Source: CAD feature listing. Evaluate the final solid. Frame: model axes, mm. Face numbers are marked on the shaded views. A direction names the side the tool comes from. Round coordinates to 2 decimals unless told otherwise and drop trailing zeros. Loops run counter-clockwise (first coordinate to the right, second up) from the corner with the lowest first, then second, coordinate; pieces in that order, holes last. Notation, with made-up numbers: (-3.75, 52.5) - (30.25, 52.5) arc R17 cw to (30.25, 63.5) - close; hole circle Ø7 at (-7, 50.25). An arc over 180 degrees is marked (long way). Write item = value, one per line. Start each with the question number.
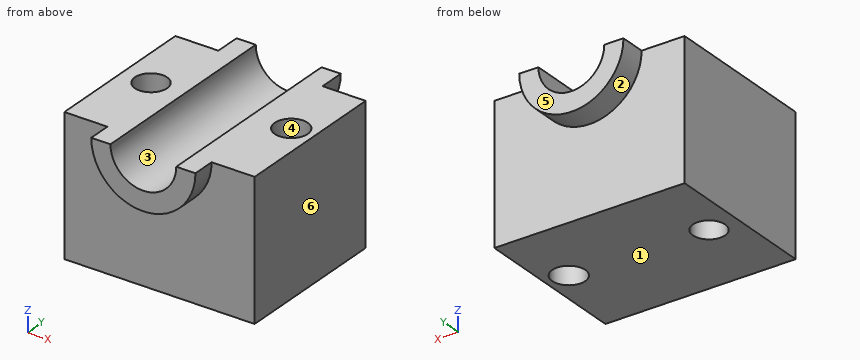
from build123d import *

# Parameters (mm, degrees)
F0_W     = 105.5908799171
F0_H     = 87.321691215
F1_DEPTH = 76.2
F3_DEPTH = 101.6
F4_DEPTH = 12.7
F5_DEPTH = 127
F6_R     = 8.9460405917
F7_DEPTH = 101.6
F6_R_2   = 9.1609397995
F8_DEPTH = 127


with BuildPart() as f1:
    # F0 (on Top) → F1 (new body)
    with BuildSketch(Plane.XY):
        with Locations((3.3811926842, 4.9695521593)):
            Rectangle(F0_W, F0_H)
    extrude(amount=F1_DEPTH)

    # F2 (on face) → F3 (join)
    with BuildSketch(Plane.XZ.offset(38.6912934482)):
        with BuildLine():
            ThreePointArc((-14.8835639872, 76.2), (3.3811926842, 57.9352433286), (21.6459493555, 76.2))
            Line((21.6459493555, 76.2), (-14.8835639872, 76.2))
        make_face()
        with BuildLine():
            ThreePointArc((-25.5366911298, 76.2), (3.3811926842, 47.282116186), (32.2990764981, 76.2))
            Line((32.2990764981, 76.2), (21.6459493555, 76.2))
            ThreePointArc((21.6459493555, 76.2), (3.3811926842, 57.9352433286), (-14.8835639872, 76.2))
            Line((-14.8835639872, 76.2), (-25.5366911298, 76.2))
        make_face()
    extrude(amount=-F3_DEPTH)

    # F2 (on face) → F4 (join)
    with BuildSketch(Plane.XZ.offset(38.6912934482)):
        with BuildLine():
            ThreePointArc((-25.5366911298, 76.2), (3.3811926842, 47.282116186), (32.2990764981, 76.2))
            Line((32.2990764981, 76.2), (21.6459493555, 76.2))
            ThreePointArc((21.6459493555, 76.2), (3.3811926842, 57.9352433286), (-14.8835639872, 76.2))
            Line((-14.8835639872, 76.2), (-25.5366911298, 76.2))
        make_face()
    extrude(amount=F4_DEPTH)

    # F5 (cut): a face of the model
    f5_faces = [f1.faces().sort_by_distance(p)[0] for p in [
        (3.3811926842, -38.6912934482, 68.4481965103),
    ]]
    extrude(f5_faces, amount=-F5_DEPTH, mode=Mode.SUBTRACT)

    # F6 (on face) → F7 (cut)
    with BuildSketch(Plane.XY.offset(76.2)):
        with Locations((-33.1366732717, 6.3863405958)):
            Circle(F6_R)
    extrude(amount=-F7_DEPTH, mode=Mode.SUBTRACT)

    # F6 (on face) → F8 (cut)
    with BuildSketch(Plane.XY.offset(76.2)):
        with Locations((43.499417603, 8.0732982606)):
            Circle(F6_R_2)
    extrude(amount=-F8_DEPTH, mode=Mode.SUBTRACT)


solid = f1.part
(1) Material intervals for line 1 along X through (y, z) = (5, 52); line 2 along X through (y, z) = (5.5, 49); line 3 along X through (y, z) = (49, 66), sorted ascending. Write a range as from..to.
(2) Access query for the marked faces 1 and 2. Directions: +Z, -Z, +X, -X, +Y, -Y. A direction counts if a zero-diameter tool reaches every point of the face in a straight line with its end or side. Return the directions, or none.
(3) Cut plane B-B (x = -33). Output: boundary loops of the cut face in (y, z), and give its area (3 significant figures).
(4) Cut plane D-D (z = 53). Output: boundary loops of the cut face in (x, y), and give its area (3 significant figures).
(5) Cut plane C-C (y = -14.5). Output: boundary loops of the cut face in (x, z).
(6) Cut plane A-A (z = 71). Output: boundary loops of the cut face in (x, y).
(7) Mould query, pull axis X, two halves, no side actions, for the marked faces 3, 4, 5 and 6. Classes: +X half, -X half, draft (parallel to the pull), parting line (faces both ways), or undercut.
(8) Pin query (flat end, axial travel): P1, Ø3, axis at x = 5.5, z = 7.5, coming from the -Y side; P2, Ø23, axis at x = -19, z = 44.5, coming from the +Y side; P3, Ø6, axis at x = -38.5, z = 51.5, coming from the +Y side. Return the tip coordinate at first contact, or that it passes through.
Solution:
q1.line_1 = -49.41..-41.97, -24.3..34.87, 52.13..56.18
q1.line_2 = -49.41..-42.04, -24.23..34.71, 52.29..56.18
q1.line_3 = -23.68..-11.77, 18.53..30.44
q2.face_1 = -Z, +X, -X, +Y, -Y
q2.face_2 = -Z, +Y
q3.outline = (-38.69, 0) - (-2.56, 0) - (-2.56, 76.2) - (-38.69, 76.2) - close; (15.33, 0) - (48.63, 0) - (48.63, 76.2) - (15.33, 76.2) - close
q3.area = 5,290 mm^2
q4.outline = (-49.41, -38.69) - (-13.88, -38.69) - (-13.88, -51.39) - (20.64, -51.39) - (20.64, -38.69) - (56.18, -38.69) - (56.18, 48.63) - (20.64, 48.63) - (20.64, 62.91) - (-13.88, 62.91) - (-13.88, 48.63) - (-49.41, 48.63) - close; hole circle Ø17.89 at (-33.14, 6.39); hole circle Ø18.32 at (43.5, 8.07)
q4.area = 9,640 mm^2
q5.outline = (-49.41, 0) - (56.18, 0) - (56.18, 76.2) - (21.65, 76.2) arc R18.26 cw to (-14.88, 76.2) - (-49.41, 76.2) - close
q6.outline = (-49.41, -38.69) - (-25.07, -38.69) - (-25.07, -51.39) - (-14.13, -51.39) - (-14.13, 62.91) - (-25.07, 62.91) - (-25.07, 48.63) - (-49.41, 48.63) - close; (20.89, -51.39) - (31.83, -51.39) - (31.83, -38.69) - (56.18, -38.69) - (56.18, 48.63) - (31.83, 48.63) - (31.83, 62.91) - (20.89, 62.91) - close; hole circle Ø17.89 at (-33.14, 6.39); hole circle Ø18.32 at (43.5, 8.07)
q7.face_3 = undercut
q7.face_4 = undercut
q7.face_5 = draft
q7.face_6 = +X half
q8.P1 = -38.69
q8.P2 = 62.91
q8.P3 = 48.63
